```python
from build123d import *

# Parameters (mm, degrees)
SKETCH1_W                      = 20
SKETCH1_H                      = 149
BOSS_EXTRUDE1_DEPTH            = 26.9
SKETCH2_W                      = 21
SKETCH2_H                      = 17.5
BOSS_EXTRUDE2_DEPTH            = 26.9
SKETCH3_W                      = 16
SKETCH3_H                      = 18.9
BOSS_EXTRUDE3_DEPTH            = 71.1
SKETCH4_R                      = 6
BOSS_EXTRUDE4_DEPTH            = 8.5
SKETCH5_R                      = 4.65
BOSS_EXTRUDE5_DEPTH            = 10
SKETCH7_W                      = 20
SKETCH7_H                      = 149
CUT_EXTRUDE1_DEPTH             = 2.8
SKETCH8_W                      = 4.5
SKETCH8_H                      = 94
CUT_EXTRUDE2_DEPTH             = 1.4
SKETCH17_R                     = 1.5
CUT_EXTRUDE3_DEPTH             = 3
SKETCH9_W                      = 20
SKETCH9_H                      = 29.8
BOSS_EXTRUDE6_DEPTH            = 4.2
SKETCH12_W                     = 20
SKETCH12_H                     = 33
BOSS_EXTRUDE7_DEPTH            = 1
SKETCH14_W                     = 11
SKETCH14_H                     = 4
BOSS_EXTRUDE8_DEPTH            = 1
SKETCH15_R                     = 1.45
BOSS_EXTRUDE9_DEPTH            = 0.5
SKETCH16_W                     = 4.5
SKETCH16_H                     = 14.5
BOSS_EXTRUDE10_DEPTH           = 1
M3X0_5_TAPPED_HOLE1_AT_2_COUNT = 2
M3X0_5_TAPPED_HOLE1_AT_2_PITCH = 16
LPATTERN1_COUNT                = 3
LPATTERN1_PITCH                = 25
FILLET1_R                      = 3
CHAMFER1_SIZE                  = 1


with BuildPart() as part:
    # Sketch1 → Boss-Extrude1 (new body)
    with BuildSketch(Plane.XY):
        with Locations((0, 74.5)):
            Rectangle(SKETCH1_W, SKETCH1_H)
    extrude(amount=-BOSS_EXTRUDE1_DEPTH)

    # Sketch2 → Boss-Extrude2 (add)
    with BuildSketch(Plane.XZ):
        with Locations((-20.5, -11.75)):
            Rectangle(SKETCH2_W, SKETCH2_H)
    extrude(amount=-BOSS_EXTRUDE2_DEPTH)

    # Sketch3 → Boss-Extrude3 (add)
    with BuildSketch(Plane(origin=(0, 26.9, 0), x_dir=(1, 0, 0), z_dir=(0, 1, 0))):
        with Locations((-20, 13.15)):
            Rectangle(SKETCH3_W, SKETCH3_H)
    extrude(amount=BOSS_EXTRUDE3_DEPTH)

    # Sketch4 → Boss-Extrude4 (add)
    with BuildSketch(Plane(origin=(0, 98, 0), x_dir=(1, 0, 0), z_dir=(0, 1, 0))):
        with Locations(Location((-20, 14.4, 0), (0, 0, 180))):
            Circle(SKETCH4_R)
    extrude(amount=BOSS_EXTRUDE4_DEPTH)

    # Sketch5 → Boss-Extrude5 (add)
    with BuildSketch(Plane(origin=(0, 106.5, 0), x_dir=(1, 0, 0), z_dir=(0, 1, 0))):
        with Locations(Location((-20, 14.4, 0), (0, 0, 180))):
            Circle(SKETCH5_R)
    extrude(amount=BOSS_EXTRUDE5_DEPTH)

    # Sketch7 → Cut-Extrude1 (cut)
    with BuildSketch(Plane.XY):
        with Locations((0, 74.5)):
            Rectangle(SKETCH7_W, SKETCH7_H)
    extrude(amount=-CUT_EXTRUDE1_DEPTH, mode=Mode.SUBTRACT)

    # Sketch8 → Cut-Extrude2 (cut)
    with BuildSketch(Plane.XY.offset(-2.8)):
        with Locations((-7.75, 102)):
            Rectangle(SKETCH8_W, SKETCH8_H)
        with Locations((7.75, 102)):
            Rectangle(SKETCH8_W, SKETCH8_H)
    extrude(amount=-CUT_EXTRUDE2_DEPTH, mode=Mode.SUBTRACT)

    # Sketch17 → Cut-Extrude3 (cut)
    with BuildSketch(Plane(origin=(0, 0, -26.9), x_dir=(-1, 0, 0), z_dir=(0, 0, -1))):
        with Locations((0, 69.5)):
            Circle(SKETCH17_R)
        with BuildLine():
            Line((1.5, 120), (1.5, 119))
            ThreePointArc((1.5, 119), (0, 117.5), (-1.5, 119))
            Line((-1.5, 119), (-1.5, 120))
            ThreePointArc((-1.5, 120), (0, 121.5), (1.5, 120))
        make_face()
    extrude(amount=-CUT_EXTRUDE3_DEPTH, mode=Mode.SUBTRACT)

    # Sketch9 → Boss-Extrude6 (add)
    with BuildSketch(Plane.XY.offset(-4.2)):
        with Locations((0, 69.9)):
            Rectangle(SKETCH9_W, SKETCH9_H)
    extrude(amount=BOSS_EXTRUDE6_DEPTH)

    # Sketch12 → Boss-Extrude7 (add)
    with BuildSketch(Plane.XY.offset(-2.8)):
        with Locations((0, 16.5)):
            Rectangle(SKETCH12_W, SKETCH12_H)
    extrude(amount=BOSS_EXTRUDE7_DEPTH)

    # Sketch14 → Boss-Extrude8 (add)
    with BuildSketch(Plane.XY.offset(-2.8)):
        with Locations((0, 147)):
            Rectangle(SKETCH14_W, SKETCH14_H)
    extrude(amount=BOSS_EXTRUDE8_DEPTH)

    # Sketch15 → Boss-Extrude9 (add)
    with BuildSketch(Plane.XY.offset(-1.8)):
        with Locations((-3, 147.5)):
            Circle(SKETCH15_R)
        with Locations((3, 147.5)):
            Circle(SKETCH15_R)
    extrude(amount=BOSS_EXTRUDE9_DEPTH)

    # Sketch16 → Boss-Extrude10 (add)
    with BuildSketch(Plane.XY.offset(-4.2)):
        with Locations((-7.75, 141.75)):
            Rectangle(SKETCH16_W, SKETCH16_H)
        with Locations((7.75, 141.75)):
            Rectangle(SKETCH16_W, SKETCH16_H)
    extrude(amount=BOSS_EXTRUDE10_DEPTH)

    # Sketch10 → M3x0.5 Tapped Hole1 (revolve, cut)
    with BuildSketch(Plane(origin=(8, 69.5, -26.9), x_dir=(0, 1, 0), z_dir=(1, 0, 0))):
        Polygon((0, 0), (0, 6.251075774), (1.25, 5.5), (1.25, 0), align=None)
    m3x0_5_tapped_hole1 = revolve(axis=Axis((8, 69.5, -33.25), (0, 0, 1)), mode=Mode.SUBTRACT)

    # M3x0.5 Tapped Hole1 at 2: M3x0.5 Tapped Hole1 ×2
    with Locations(*[(-i * M3X0_5_TAPPED_HOLE1_AT_2_PITCH, 0, 0) for i in range(1, M3X0_5_TAPPED_HOLE1_AT_2_COUNT)]):
        add(m3x0_5_tapped_hole1, mode=Mode.SUBTRACT)

    # LPattern1: M3x0.5 Tapped Hole1 ×3
    with Locations(*[(0, i * LPATTERN1_PITCH, 0) for i in range(1, LPATTERN1_COUNT)]):
        add(m3x0_5_tapped_hole1, mode=Mode.SUBTRACT)

    # LPattern1 copy 1 sketch → LPattern1 copy 1 (revolve, cut)
    with BuildSketch(Plane(origin=(-8, 94.5, -26.9), x_dir=(0, 1, 0), z_dir=(1, 0, 0))):
        Polygon((0, 0), (0, 6.251075774), (1.25, 5.5), (1.25, 0), align=None)
    revolve(axis=Axis((-8, 94.5, -33.25), (0, 0, 1)), mode=Mode.SUBTRACT)

    # LPattern1 copy 2 sketch → LPattern1 copy 2 (revolve, cut)
    with BuildSketch(Plane(origin=(-8, 119.5, -26.9), x_dir=(0, 1, 0), z_dir=(1, 0, 0))):
        Polygon((0, 0), (0, 6.251075774), (1.25, 5.5), (1.25, 0), align=None)
    revolve(axis=Axis((-8, 119.5, -33.25), (0, 0, 1)), mode=Mode.SUBTRACT)

    # Fillet1
    # the kernel refuses this fillet: 3 mm, written as the material it takes off along each edge
    with BuildSketch(Plane(origin=(-17.483314774, 55, 0), x_dir=(0, 1, 0), z_dir=(1, 0, 0))) as fillet1_piece_1:
        with BuildLine():
            CenterArc((2.993325909, -3), FILLET1_R, 90, 86.177446271)
            Line((0, -2.8), (0, 0))
            Line((0, 0), (2.993325909, 0))
        make_face()
    extrude(amount=34.966629547, mode=Mode.SUBTRACT)
    with BuildSketch(Plane(origin=(17.5, 84.8, 0), x_dir=(0, 0, -1), z_dir=(-1, 0, 0))) as fillet1_piece_2_section:
        with BuildLine():
            CenterArc((FILLET1_R, FILLET1_R), FILLET1_R, 180, 90)
            Line((0, FILLET1_R), (0, 0))
            Line((0, 0), (FILLET1_R, 0))
        make_face()
    fillet1_piece_2 = extrude(amount=35, mode=Mode.PRIVATE)
    fillet1_piece_2 = split(fillet1_piece_2, bisect_by=Plane(origin=(5.5, 84.8, 0), z_dir=(1, 0, 0)), keep=Keep.TOP, mode=Mode.PRIVATE)
    add(fillet1_piece_2, mode=Mode.SUBTRACT)
    with BuildSketch(Plane(origin=(17.5, 84.8, 0), x_dir=(0, 0, -1), z_dir=(-1, 0, 0))) as fillet1_piece_3_section:
        with BuildLine():
            CenterArc((FILLET1_R, FILLET1_R), FILLET1_R, 180, 90)
            Line((0, FILLET1_R), (0, 0))
            Line((0, 0), (FILLET1_R, 0))
        make_face()
    fillet1_piece_3 = extrude(amount=35, mode=Mode.PRIVATE)
    fillet1_piece_3 = split(fillet1_piece_3, bisect_by=Plane(origin=(17.5, 84.8, -2.8), z_dir=(0, 0, 1)), keep=Keep.TOP, mode=Mode.PRIVATE)
    add(fillet1_piece_3, mode=Mode.SUBTRACT)
    with BuildSketch(Plane(origin=(17.5, 84.8, 0), x_dir=(0, 0, -1), z_dir=(-1, 0, 0))) as fillet1_piece_4_section:
        with BuildLine():
            CenterArc((FILLET1_R, FILLET1_R), FILLET1_R, 180, 90)
            Line((0, FILLET1_R), (0, 0))
            Line((0, 0), (FILLET1_R, 0))
        make_face()
    fillet1_piece_4 = extrude(amount=35, mode=Mode.PRIVATE)
    fillet1_piece_4 = split(fillet1_piece_4, bisect_by=Plane(origin=(-5.5, 84.8, 0), z_dir=(-1, 0, 0)), keep=Keep.TOP, mode=Mode.PRIVATE)
    add(fillet1_piece_4, mode=Mode.SUBTRACT)

    # Chamfer1
    chamfer1_edges = [part.edges().sort_by_distance(p)[0] for p in [
        (-28, 98, -13.15),
        (-20, 98, -3.7),
        (-12, 98, -13.15),
        (-20, 98, -22.6),
    ]]
    chamfer(chamfer1_edges, length=CHAMFER1_SIZE)


solid = part.part
```
Design review of the part built by this model. Coordinates are the model's own, in mm. A direction names the side the tool comes from. Give positions to 0.01 mm unless a question says otherwise; leave off trailing zeros. Order: outer loops, then holes, each group sorted by start corner. A loop starts at its lowest first (then second) coordinate and runs counter-clockwise, first axis right, second up. Notation, with made-up numbers: (-15, -2) -> (-8, -2) arc R28 cw to (-8, 28) -> close; hole circle Ø11 at (78.5, 30.5). An arc over 180 degrees is marked (long way). Write each question's results on one line, items separated by ' | '. Start each with the question number.
Q1. Wall thickness on L1, parallel to X at y = 69.5, z = -23.35; L2, parallel to X at y = 119.5, z = -24.9; L3, parallel to Y at x = 8, z = -24.55: over which ranges is each line inside the solid? List them lowest first. Write a range as from..to.
Q2. Add section B-B on x = 3. Give the boundary of the cut face in (y, z), and give its area (3 significant figures).
Q3. Mouldability with a two-part tool opening along Y and no side actions: class faces 1 (the flat face through (-8, 110, -4.2)), 2 (the flat face through (-22, 106.5, -19)), 3 (the flat face through (-31, 13, -12)), 4 (the flat face through (-5.5, 109, -4)) as +Y half, -Y half, draft (parallel to the pull), parting line (faces both ways), or undercut.
Q4. Machinability: for faces 5 (the flat face through (-20, 98, -8)), 6 (the flat face through (8, 142, -3.2)), 7 (the cylindrical face through (8.479, 120.655, -24.188)), 8 (the flat face through (8, 110, -4.2)), 9 (the cylindrical face through (-0.14, 55.967, -0.788)), which of the approach directions +Z, -Z, +X, -X, +Y, -Y give a long, thin tool a straight path to every point of the face, cutting with its end or side? Answer none if there is none.
Q5. Add section D-D on y = 147.5. Give the boundary of the cut face in (x, z), and give its area (3 significant figures).
Q6. Add section A-A on y = 21. Give the boundary of the cut face in (x, z), and give its area (4 significant figures).
Q7. Add section C-C on z = -14.4. Give the boundary of the cut face in (x, y), and give its area (3 significant figures).
Q8. For pin 1 (4 mm diameter, centred on x = -10.5, y = 42.5, fed in from +Z); pin 2 (17.5 mm diameter, centred on x = -24, y = 54.5, fed in from +Z); pin 3 (1.5 mm diameter, centred on x = -8, y = 94.5, fed in from -Z), all flat-tipped, find the tip position at first contact; note any pin that passes through.
Found:
1) L1: x = -10..-9.25, -6.75..6.75, 9.25..10 | L2: x = -10..-9.25, -6.75..-1.5, 1.5..6.75, 9.25..10 | L3: y = 0..68.25, 70.75..93.25, 95.75..118.25, 120.75..149
2) outline: (0, -26.9) -> (149, -26.9) -> (149, -1.8) -> (148.95, -1.8) -> (148.95, -1.3) -> (146.05, -1.3) -> (146.05, -1.8) -> (145, -1.8) -> (145, -2.8) -> (84.79, -2.8) arc R3 ccw to (81.8, 0) -> (57.99, 0) arc R3 ccw to (55, -2.8) -> (33, -2.8) -> (33, -1.8) -> (0, -1.8) -> close | area: 3,710 mm2
3) face 1: undercut | face 2: +Y half | face 3: draft | face 4: undercut
4) face 5: +Y | face 6: +Z, +X, +Y | face 7: -Z | face 8: +Z, +X | face 9: +Z, +X, -X
5) outline: (-10, -26.9) -> (10, -26.9) -> (10, -3.2) -> (5.5, -3.2) -> (5.5, -1.8) -> (4.45, -1.8) -> (4.45, -1.3) -> (1.55, -1.3) -> (1.55, -1.8) -> (-1.55, -1.8) -> (-1.55, -1.3) -> (-4.45, -1.3) -> (-4.45, -1.8) -> (-5.5, -1.8) -> (-5.5, -3.2) -> (-10, -3.2) -> close | area: 492 mm2
6) outline: (-31, -20.5) -> (-10, -20.5) -> (-10, -26.9) -> (10, -26.9) -> (10, -1.8) -> (-10, -1.8) -> (-10, -3) -> (-31, -3) -> close | area: 869.5 mm2
7) outline: (-31, 0) -> (10, 0) -> (10, 149) -> (-10, 149) -> (-10, 26.9) -> (-12, 26.9) -> (-12, 97) -> (-13, 98) -> (-14, 98) -> (-14, 106.5) -> (-15.35, 106.5) -> (-15.35, 116.5) -> (-24.65, 116.5) -> (-24.65, 106.5) -> (-26, 106.5) -> (-26, 98) -> (-27, 98) -> (-28, 97) -> (-28, 26.9) -> (-31, 26.9) -> close | area: 4,880 mm2
8) pin 1: stops at z = -2.8 | pin 2: stops at z = -3.7 | pin 3: stops at z = -21.1
